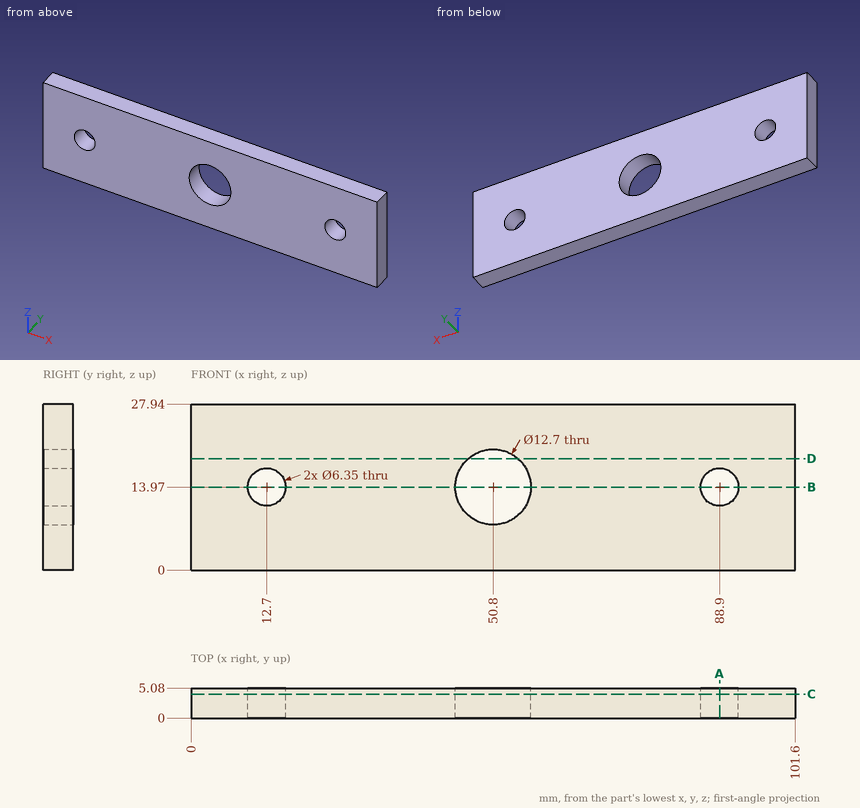
Could you check a few things on this drawing? It's one solid part, dimensions in mm from its lowest x, y, z. Coordinates: 2 decimals unless noted, no trailing zeros. Order: outer loops, then holes, each group sorted by start corner. A loop starts at its lowest first (then second) coordinate and runs counter-clockwise, first axis right, second up.
1. If we section it at C-C (y = 4.05): Please give me the cut outline in (x, z) (3 decimals), then the cut area to 3 significant figures.
2. I need wall thicknesses on line 1 (Z direction, x = 50.8, y = 3.35); line 2 (Z direction, x = 88.9, y = 2.2) (3 decimals); line 3 (X direction, y = 0.5, z = 16). Which ranges of each line are inside material? Lowest first, please.
3. If we section it at A-A (x = 88.9): Please give me the cut outline in (y, z) (3 decimals), then the cut area to 3 significant figures.
4. If we section it at D-D (z = 18.75): Please give me the cut outline in (x, y).
5. If we section it at B-B (z = 13.97): Please give me the cut outline in (x, y) (3 decimals), then the cut area to 3 significant figures.
Entries:
1. outline: (0, 0) - (101.6, 0) - (101.6, 27.94) - (0, 27.94) - close; hole circle Ø6.35 at (12.7, 13.97); hole circle Ø12.7 at (50.8, 13.97); hole circle Ø6.35 at (88.9, 13.97)
1. area: 2,650 mm2
2. line 1: z = 0 to 7.62, 20.32 to 27.94
2. line 2: z = 0 to 10.795, 17.145 to 27.94
2. line 3: x = 0 to 10.26, 15.14 to 44.78, 56.82 to 86.46, 91.34 to 101.6
3. outline: (0, 0) - (5.08, 0) - (5.08, 10.795) - (0, 10.795) - close; (0, 17.145) - (5.08, 17.145) - (5.08, 27.94) - (0, 27.94) - close
3. area: 110 mm2
4. outline: (0, 0) - (46.62, 0) - (46.62, 5.08) - (0, 5.08) - close; (54.98, 0) - (101.6, 0) - (101.6, 5.08) - (54.98, 5.08) - close
5. outline: (0, 0) - (9.525, 0) - (9.525, 5.08) - (0, 5.08) - close; (15.875, 0) - (44.45, 0) - (44.45, 5.08) - (15.875, 5.08) - close; (57.15, 0) - (85.725, 0) - (85.725, 5.08) - (57.15, 5.08) - close; (92.075, 0) - (101.6, 0) - (101.6, 5.08) - (92.075, 5.08) - close
5. area: 387 mm2
